from build123d import *

# Parameters (mm, degrees)
F0_W      = 1244.6
F0_H      = 762
F1_DEPTH  = 165.1
F3_DEPTH  = 152.4
F5_DEPTH  = 355.6
F7_DEPTH  = 355.6
F9_DEPTH  = 152.4
F10_R     = 12.7
F11_DEPTH = 50.8
F12_R     = 12.7
F13_DEPTH = 165.101
F15_R     = 25.4
F16_DEPTH = 25.4
F17_R     = 25.4
F18_DEPTH = 165.101


with BuildPart() as f1:
    # F0 (on Top) → F1 (new body)
    with BuildSketch(Plane.XY):
        with Locations((622.3, 381)):
            Rectangle(F0_W, F0_H)
    extrude(amount=-F1_DEPTH)

    # F2 (on face) → F3 (cut)
    with BuildSketch(Plane.XZ):
        Polygon((457.2, -25.4), (444.5, -25.4), (444.5, -50.8), (495.3, -50.8), (495.3, -25.4), (482.6, -25.4), (482.6, 0), (457.2, 0), align=None)
        Polygon((635, 0), (609.6, 0), (609.6, -25.4), (596.9, -25.4), (596.9, -50.8), (647.7, -50.8), (647.7, -25.4), (635, -25.4), align=None)
        Polygon((787.4, 0), (762, 0), (762, -25.4), (749.3, -25.4), (749.3, -50.8), (800.1, -50.8), (800.1, -25.4), (787.4, -25.4), align=None)
    extrude(amount=-F3_DEPTH, mode=Mode.SUBTRACT)

    # F4 (on face) → F5 (cut)
    with BuildSketch(Plane.YZ.offset(1244.6)):
        Polygon((241.3, 0), (215.9, 0), (215.9, -25.4), (203.2, -25.4), (203.2, -50.8), (254, -50.8), (254, -25.4), (241.3, -25.4), align=None)
        Polygon((393.7, 0), (368.3, 0), (368.3, -25.4), (355.6, -25.4), (355.6, -50.8), (406.4, -50.8), (406.4, -25.4), (393.7, -25.4), align=None)
        Polygon((546.1, 0), (520.7, 0), (520.7, -25.4), (508, -25.4), (508, -50.8), (558.8, -50.8), (558.8, -25.4), (546.1, -25.4), align=None)
    extrude(amount=-F5_DEPTH, mode=Mode.SUBTRACT)

    # F6 (on face) → F7 (cut)
    with BuildSketch(Plane(origin=(0, 0, 0), x_dir=(0, -1, 0), z_dir=(-1, 0, 0))):
        Polygon((-520.7, 0), (-546.1, 0), (-546.1, -25.4), (-558.8, -25.4), (-558.8, -50.8), (-508, -50.8), (-508, -25.4), (-520.7, -25.4), align=None)
        Polygon((-368.3, 0), (-393.7, 0), (-393.7, -25.4), (-406.4, -25.4), (-406.4, -50.8), (-355.6, -50.8), (-355.6, -25.4), (-368.3, -25.4), align=None)
        Polygon((-215.9, 0), (-241.3, 0), (-241.3, -25.4), (-254, -25.4), (-254, -50.8), (-203.2, -50.8), (-203.2, -25.4), (-215.9, -25.4), align=None)
    extrude(amount=-F7_DEPTH, mode=Mode.SUBTRACT)

    # F8 (on face) → F9 (cut)
    with BuildSketch(Plane(origin=(0, 762, 0), x_dir=(-1, 0, 0), z_dir=(0, 1, 0))):
        Polygon((-762, 0), (-787.4, 0), (-787.4, -25.4), (-800.1, -25.4), (-800.1, -50.8), (-749.3, -50.8), (-749.3, -25.4), (-762, -25.4), align=None)
        Polygon((-609.6, 0), (-635, 0), (-635, -25.4), (-647.7, -25.4), (-647.7, -50.8), (-596.9, -50.8), (-596.9, -25.4), (-609.6, -25.4), align=None)
        Polygon((-457.2, 0), (-482.6, 0), (-482.6, -25.4), (-495.3, -25.4), (-495.3, -50.8), (-444.5, -50.8), (-444.5, -25.4), (-457.2, -25.4), align=None)
    extrude(amount=-F9_DEPTH, mode=Mode.SUBTRACT)

    # F10 (on face) → F11 (cut)
    with BuildSketch(Plane.XY):
        with BuildLine():
            ThreePointArc((482.6, 609.6), (469.9, 622.3), (457.2, 609.6))
            Line((457.2, 609.6), (482.6, 609.6))
        make_face()
        with BuildLine():
            Line((482.6, 609.6), (457.2, 609.6))
            ThreePointArc((457.2, 609.6), (469.9, 596.9), (482.6, 609.6))
        make_face()
        with BuildLine():
            ThreePointArc((635, 609.6), (622.3, 622.3), (609.6, 609.6))
            Line((609.6, 609.6), (635, 609.6))
        make_face()
        with BuildLine():
            Line((635, 609.6), (609.6, 609.6))
            ThreePointArc((609.6, 609.6), (622.3, 596.9), (635, 609.6))
        make_face()
        with BuildLine():
            ThreePointArc((787.4, 609.6), (774.7, 622.3), (762, 609.6))
            Line((762, 609.6), (787.4, 609.6))
        make_face()
        with BuildLine():
            Line((787.4, 609.6), (762, 609.6))
            ThreePointArc((762, 609.6), (774.7, 596.9), (787.4, 609.6))
        make_face()
        with BuildLine():
            ThreePointArc((889, 546.1), (876.3, 533.4), (889, 520.7))
            Line((889, 520.7), (889, 546.1))
        make_face()
        with BuildLine():
            Line((889, 546.1), (889, 520.7))
            ThreePointArc((889, 520.7), (897.9802561211, 524.4197438789), (901.7, 533.4))
            ThreePointArc((901.7, 533.4), (897.9802561211, 542.3802561211), (889, 546.1))
        make_face()
        with BuildLine():
            ThreePointArc((889, 393.7), (876.3, 381), (889, 368.3))
            Line((889, 368.3), (889, 393.7))
        make_face()
        with BuildLine():
            Line((889, 393.7), (889, 368.3))
            ThreePointArc((889, 368.3), (897.9802561211, 372.0197438789), (901.7, 381))
            ThreePointArc((901.7, 381), (897.9802561211, 389.9802561211), (889, 393.7))
        make_face()
        with BuildLine():
            ThreePointArc((889, 241.3), (876.3, 228.6), (889, 215.9))
            Line((889, 215.9), (889, 241.3))
        make_face()
        with BuildLine():
            Line((889, 241.3), (889, 215.9))
            ThreePointArc((889, 215.9), (897.9802561211, 219.6197438789), (901.7, 228.6))
            ThreePointArc((901.7, 228.6), (897.9802561211, 237.5802561211), (889, 241.3))
        make_face()
        with BuildLine():
            ThreePointArc((355.6, 393.7), (342.9, 381), (355.6, 368.3))
            Line((355.6, 368.3), (355.6, 393.7))
        make_face()
        with BuildLine():
            Line((355.6, 393.7), (355.6, 368.3))
            ThreePointArc((355.6, 368.3), (364.5802561211, 372.0197438789), (368.3, 381))
            ThreePointArc((368.3, 381), (364.5802561211, 389.9802561211), (355.6, 393.7))
        make_face()
        with BuildLine():
            ThreePointArc((482.6, 152.4), (469.9, 165.1), (457.2, 152.4))
            Line((457.2, 152.4), (482.6, 152.4))
        make_face()
        with BuildLine():
            Line((482.6, 152.4), (457.2, 152.4))
            ThreePointArc((457.2, 152.4), (469.9, 139.7), (482.6, 152.4))
        make_face()
        with BuildLine():
            ThreePointArc((635, 152.4), (622.3, 165.1), (609.6, 152.4))
            Line((609.6, 152.4), (635, 152.4))
        make_face()
        with BuildLine():
            Line((635, 152.4), (609.6, 152.4))
            ThreePointArc((609.6, 152.4), (622.3, 139.7), (635, 152.4))
        make_face()
        with BuildLine():
            ThreePointArc((787.4, 152.4), (774.7, 165.1), (762, 152.4))
            Line((762, 152.4), (787.4, 152.4))
        make_face()
        with BuildLine():
            Line((787.4, 152.4), (762, 152.4))
            ThreePointArc((762, 152.4), (774.7, 139.7), (787.4, 152.4))
        make_face()
        with Locations((355.6, 533.4)):
            Circle(F10_R)
        with Locations((355.6, 228.6)):
            Circle(F10_R)
    extrude(amount=-F11_DEPTH, mode=Mode.SUBTRACT)

    # F12 (on face) → F13 (cut, through all)
    with BuildSketch(Plane.XY):
        with BuildLine():
            ThreePointArc((419.1, 495.3), (431.8, 482.6), (444.5, 495.3))
            ThreePointArc((444.5, 495.3), (431.8, 508), (419.1, 495.3))
        make_face()
        with Locations((508, 495.3)):
            Circle(F12_R)
        with Locations((584.2, 495.3)):
            Circle(F12_R)
        with Locations((660.4, 495.3)):
            Circle(F12_R)
        with Locations((736.6, 495.3)):
            Circle(F12_R)
        with BuildLine():
            Line((812.8, 495.3), (825.5, 495.3))
            ThreePointArc((825.5, 495.3), (821.7802561211, 504.2802561211), (812.8, 508))
            Line((812.8, 508), (812.8, 495.3))
        make_face()
        with BuildLine():
            ThreePointArc((812.8, 508), (803.8197438789, 486.3197438789), (825.5, 495.3))
            Line((825.5, 495.3), (812.8, 495.3))
            Line((812.8, 495.3), (812.8, 508))
        make_face()
        with Locations((431.8, 419.1)):
            Circle(F12_R)
        with Locations((508, 419.1)):
            Circle(F12_R)
        with Locations((584.2, 419.1)):
            Circle(F12_R)
        with Locations((660.4, 419.1)):
            Circle(F12_R)
        with Locations((736.6, 419.1)):
            Circle(F12_R)
        with Locations((812.8, 419.1)):
            Circle(F12_R)
        with Locations((431.8, 342.9)):
            Circle(F12_R)
        with Locations((508, 342.9)):
            Circle(F12_R)
        with Locations((584.2, 342.9)):
            Circle(F12_R)
        with Locations((660.4, 342.9)):
            Circle(F12_R)
        with Locations((736.6, 342.9)):
            Circle(F12_R)
        with Locations((812.8, 342.9)):
            Circle(F12_R)
        with Locations((431.8, 266.7)):
            Circle(F12_R)
        with Locations((508, 266.7)):
            Circle(F12_R)
        with Locations((584.2, 266.7)):
            Circle(F12_R)
        with Locations((660.4, 266.7)):
            Circle(F12_R)
        with Locations((736.6, 266.7)):
            Circle(F12_R)
        with BuildLine():
            ThreePointArc((812.8, 254), (821.7802561211, 257.7197438789), (825.5, 266.7))
            ThreePointArc((825.5, 266.7), (803.8197438789, 275.6802561211), (812.8, 254))
        make_face()
    extrude(amount=-F13_DEPTH, mode=Mode.SUBTRACT)

    # F15 (on offset) → F16 (cut)
    with BuildSketch(Plane.XY.offset(-25.4)):
        with BuildLine():
            ThreePointArc((749.3, 152.4), (774.7, 127), (800.1, 152.4))
            ThreePointArc((800.1, 152.4), (774.7, 177.8), (749.3, 152.4))
        make_face()
        with Locations((622.3, 152.4)):
            Circle(F15_R)
        with Locations((469.9, 152.4)):
            Circle(F15_R)
        with Locations((355.6, 381)):
            Circle(F15_R)
        with Locations((889, 381)):
            Circle(F15_R)
        with Locations((889, 228.6)):
            Circle(F15_R)
        with Locations((774.7, 609.6)):
            Circle(F15_R)
        with Locations((622.3, 609.6)):
            Circle(F15_R)
        with Locations((469.9, 609.6)):
            Circle(F15_R)
        with Locations((889, 533.4)):
            Circle(F15_R)
        with Locations((355.6, 228.6)):
            Circle(F15_R)
        with Locations((355.6, 533.4)):
            Circle(F15_R)
    extrude(amount=-F16_DEPTH, mode=Mode.SUBTRACT)

    # F17 (on face) → F18 (cut, through all)
    with BuildSketch(Plane.XY):
        with Locations((127, 622.3)):
            Circle(F17_R)
        with Locations((1117.6, 622.3)):
            Circle(F17_R)
        with Locations((127, 139.7)):
            Circle(F17_R)
        with Locations((1117.6, 139.7)):
            Circle(F17_R)
    extrude(amount=-F18_DEPTH, mode=Mode.SUBTRACT)


solid = f1.part
Geometry check sheet. Reference: the model listing, model coordinates, mm. A direction names the side the tool comes from. Round coordinates to 2 decimals unless told otherwise and drop trailing zeros. Order: outer loops, then holes, each group sorted by start corner. A loop starts at its lowest first (then second) coordinate and runs counter-clockwise, first axis right, second up. Notation, with made-up numbers: M 48,71.5 L 78,71.5 A12 cw 78,90.5 Z; hole C 50,-18.75 d8. An arc over 180 degrees is marked long. Answer in a Markdown table with one row per item.
(1) Go/stop test with flat-tipped pins: P1, Ø4, axis at x = 1088, y = 112.5, coming from the +Z side; P2, Ø3, axis at x = 468, y = 681, coming from the +Z side. Record where each tip stops, or that it passes through.
Responses:
| item | result |
|---|---|
| P1 | stops at z = 0 |
| P2 | stops at z = -50.8 |
(2) Scan lines: probe 1 along Y at (x, z) = (431.8, -38); probe 2 along Y at (x, z) = (1013.5, -10.5); probe 3 along X at (y, z) = (68.5, -42). Record each from-to range of solid material in increasing order. Write a range as from..to.
Responses:
| item | result |
|---|---|
| probe 1 | y = 0..254, 279.4..330.2, 355.6..406.4, 431.8..482.6, 508..762 |
| probe 2 | y = 0..215.9, 241.3..368.3, 393.7..520.7, 546.1..762 |
| probe 3 | x = 0..444.5, 495.3..596.9, 647.7..749.3, 800.1..1244.6 |
(3) Tool access check on faces 1 (the face through (749.3, 75, -38)), 2 (the face through (1069, 508, -38)), 3 (the face through (775, 674, -50.8)), 4 (the face through (175, 520.7, -13)). Record the directions out of +Z, -Z, +X, -X, +Y, -Y that give a thin tool (end or side, any length) a straight path to the whole face; none if there is none.
Responses:
| item | result |
|---|---|
| face 1 | -Y |
| face 2 | +X |
| face 3 | +Y |
| face 4 | +Z, -X |
(4) Sectioned sample at C-C, the plane y = 228.6. Record the cut outline in (x, z), and give its area (3 significant figures).
Responses:
| item | result |
|---|---|
| outline | M 0,-165.1 L 1244.6,-165.1 L 1244.6,-50.8 L 863.6,-50.8 L 863.6,-25.4 L 876.3,-25.4 L 876.3,0 L 368.3,0 L 368.3,-25.4 L 381,-25.4 L 381,-50.8 L 0,-50.8 Z |
| area | 167,000 mm² |
(5) Sectioned sample at A-A, the plane x = 736.6. Record the cut outline in (y, z), and give its area (3 significant figures).
Responses:
| item | result |
|---|---|
| outline | M 0,-165.1 L 254,-165.1 L 254,0 L 0,0 Z; M 279.4,-165.1 L 330.2,-165.1 L 330.2,0 L 279.4,0 Z; M 355.6,-165.1 L 406.4,-165.1 L 406.4,0 L 355.6,0 Z; M 431.8,-165.1 L 482.6,-165.1 L 482.6,0 L 431.8,0 Z; M 508,-165.1 L 762,-165.1 L 762,0 L 508,0 Z |
| area | 109,000 mm² |
(6) Sectioned sample at B-B, the plane z = -109. State how many separate pieces and enclosed holes the cut face has, and give its area (3 significant figures).
Responses:
| item | result |
|---|---|
| separate pieces | 1 |
| enclosed holes | 28 |
| area | 928,000 mm² |
(7) Draft check along Y on faces 5 (the face through (774.141, 584.206, -37.922)), 6 (the face through (175, 508, -38)), 7 (the face through (758, 88, -25.4)). Enter one of: released by +Y, released by -Y, zero draft, split by the parting line, or undercut.
Responses:
| item | result |
|---|---|
| face 5 | released by +Y |
| face 6 | undercut |
| face 7 | zero draft |
